The listing builds one solid part. Answer for the finished solid, in the listing's coordinates (mm). Face numbers are marked on the shaded views. A direction names the side the tool comes from. Coordinates: 2 decimals unless noted, no trailing zeros. Order: outer loops, then holes, each group sorted by start corner. A loop starts at its lowest first (then second) coordinate and runs counter-clockwise, first axis right, second up. Notation, with made-up numbers: M 12.5,-22 L 64.5,-22 A22 cw 64.5,-2 Z; hole C -36.5,-31.75 d7. An arc over 180 degrees is marked long. One line per item, written item: value. Start each with the question number.
Q1. Determine the mould class of the marked faces 5, 6 and 7 for opening direction X: pulls with the +X half, pulls with the -X half, needs draft (parallel to the pull), parting line crosses it, or undercut.
Q2. The part is cut by section B-B on x = 0. Give the vertices of the cut face in (y, z).
Q3. For the marked faces 1, 2, 3 and 4, determine the directions among +Z, -Z, +X, -X, +Y, -Y from which every point of the face is accessible in a straight line to the end or side of a thin tool.
Q4. The part is cut by section C-C on z = -15. Give the vertices of the cut face in (x, y), then the cut area to 3 significant figures.
Q5. The part is cut by section D-D on y = 29.5. Give the vertices of the cut face in (x, z).
Q6. Each of these flat-tipped pins is pushed along its axis until it touches: pin 1 Ø2 at (x, z) = (5, -11) entering from +Y; pin 2 Ø12 at (x, z) = (23, -5.5) entering from +Y; pin 3 Ø20 at (x, y) = (-17.5, 25) entering from +Z; pin 4 Ø8.5 at (x, z) = (0, -15) entering from +Y. Where does it stop, or does it pass through?
Q7. Straight lines are drawn through the part: line 1 along X through (y, z) = (13, -15); line 2 along X through (y, z) = (5.75, 12); line 3 along X through (y, z) = (6, -14). For each, find the intervals that lie inside material, in ascending order. Write a range as [from, to].
Q8. The part is cut by section A-A on y = 11. Give the vertices of the cut face in (x, z).
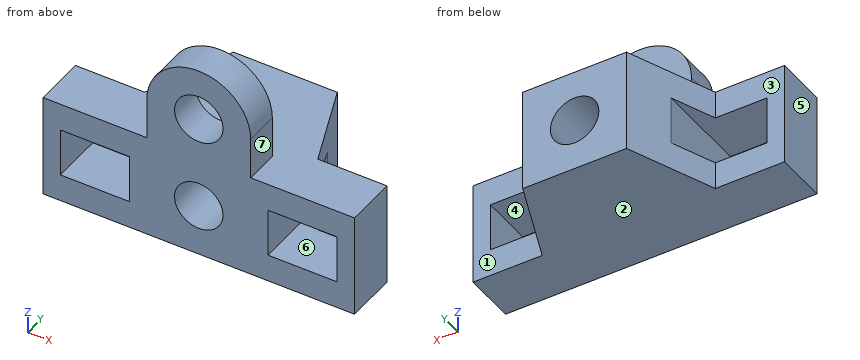
```python
from build123d import *

# Parameters (mm, degrees)
BOSS_EXTRUDE1_DEPTH     = 30
CUT_EXTRUDE1_DEPTH      = 68.268120235
CUT_EXTRUDE1_DEPTH_BACK = 68.268120235
SKETCH3_W               = 20
SKETCH3_H               = 14
CUT_EXTRUDE2_DEPTH      = 68.268120235
CUT_EXTRUDE2_DEPTH_BACK = 68.268120235
SKETCH4_R               = 7
SKETCH5_R               = 7
BOSS_EXTRUDE3_DEPTH     = 10


with BuildPart() as part:
    # Sketch2 → Boss-Extrude1 (new body)
    with BuildSketch(Plane.XY):
        Polygon((-45, 0), (45, 0), (45, 15), (25, 15), (15, 40), (-15, 40), (-25, 15), (-45, 15), align=None)
    extrude(amount=-BOSS_EXTRUDE1_DEPTH)

    # Sketch3 → Cut-Extrude1 (cut, two sides: drawn at the far end of the back side and taken through both)
    with BuildSketch(Plane(origin=(0, 0, 0), x_dir=(1, 0, 0), z_dir=(0, 1, 0)).offset(-CUT_EXTRUDE1_DEPTH_BACK)):
        with Locations((-30, 15)):
            Rectangle(SKETCH3_W, SKETCH3_H)
        with Locations((30, 15)):
            Rectangle(SKETCH3_W, SKETCH3_H)
    extrude(amount=CUT_EXTRUDE1_DEPTH + CUT_EXTRUDE1_DEPTH_BACK, mode=Mode.SUBTRACT)

    # Sketch4 → Cut-Extrude2 (cut, two sides: drawn at the far end of the back side and taken through both)
    with BuildSketch(Plane(origin=(0, 0, 0), x_dir=(1, 0, 0), z_dir=(0, 1, 0)).offset(-CUT_EXTRUDE2_DEPTH_BACK)):
        with Locations(Location((0, 15, 0), (0, 0, 90))):
            Circle(SKETCH4_R)
    extrude(amount=CUT_EXTRUDE2_DEPTH + CUT_EXTRUDE2_DEPTH_BACK, mode=Mode.SUBTRACT)

    # Sketch5 → Boss-Extrude3 (add)
    with BuildSketch(Plane(origin=(0, 0, 0), x_dir=(1, 0, 0), z_dir=(0, 1, 0))):
        with BuildLine():
            Line((-15, 0), (-15, -12))
            ThreePointArc((-15, -12), (0, -27), (15, -12))
            Line((15, -12), (15, 0))
            Line((15, 0), (-15, 0))
        make_face()
        with Locations(Location((0, -12, 0), (0, 0, 270))):
            Circle(SKETCH5_R, mode=Mode.SUBTRACT)
    extrude(amount=BOSS_EXTRUDE3_DEPTH)


solid = part.part
```
Output:
1. face 5: pulls with the -X half
1. face 6: undercut
1. face 7: pulls with the +X half
2. outline: M 0,-30 L 40,-30 L 40,-22 L 0,-22 Z; M 0,-8 L 40,-8 L 40,0 L 10,0 L 10,5 L 0,5 Z; M 0,19 L 10,19 L 10,27 L 0,27 Z
3. face 1: +Z, -Z, +X, +Y
3. face 2: -Z, +X, -X, +Y, -Y
3. face 3: +Z, -Z, -X, +Y
3. face 4: +Y, -Y
4. outline: M -45,0 L -40,0 L -40,15 L -45,15 Z; M -20,0 L -7,0 L -7,40 L -15,40 L -20,27.5 Z; M 7,0 L 20,0 L 20,27.5 L 15,40 L 7,40 Z; M 40,0 L 45,0 L 45,15 L 40,15 Z
4. area: 1,130 mm^2
5. outline: M -19.2,-30 L 19.2,-30 L 19.2,0 L -19.2,0 Z; hole C 0,-15 d14
6. pin 1: stops at y = 40
6. pin 2: stops at y = 35
6. pin 3: stops at z = 0
6. pin 4: passes through
7. line 1: x = [-45, -40], [-20, -7], [7, 20], [40, 45]
7. line 2: x = [-15, -7], [7, 15]
7. line 3: x = [-45, -40], [-20, -6.93], [6.93, 20], [40, 45]
8. outline: M -45,-30 L 45,-30 L 45,0 L -45,0 Z; hole M -40,-22 L -20,-22 L -20,-8 L -40,-8 Z; hole C 0,-15 d14; hole M 20,-22 L 40,-22 L 40,-8 L 20,-8 Z
